For this review, take the finished solid that the model builds, in its own axes (mm). A direction names the side the tool comes from. Round coordinates to 2 decimals unless told otherwise and drop trailing zeros.
from build123d import *

# Parameters (mm, degrees)
SALIENTE_EXTRUIR1_DEPTH = 5.5
CROQUIS3_W              = 12.5
CROQUIS3_H              = 5.5
SALIENTE_EXTRUIR2_DEPTH = 25
CROQUIS6_R              = 0.88
CORTAR_EXTRUIR3_DEPTH   = 1
CORTAR_EXTRUIR4_DEPTH   = 5.75
CROQUIS7_W              = 3.3125
CROQUIS7_H              = 5.5
SALIENTE_EXTRUIR3_DEPTH = 5
SALIENTE_EXTRUIR6_DEPTH = 5.5


with BuildPart() as part:
    # Croquis2 → Saliente-Extruir1 (new body)
    with BuildSketch(Plane(origin=(0, 0, 0), x_dir=(1, 0, 0), z_dir=(0, 1, 0))):
        with BuildLine():
            Line((0, 0), (0, 12.5))
            Line((0, 12.5), (90, 36.615427319))
            add(Edge.make_bspline(
                [(0, 0), (0.391394635, 0.015775005), (1.186974035, 0.048775969), (2.973718865, 0.125104104), (4.540088904, 0.200260299), (6.566615662, 0.300718996), (8.325276336, 0.397659311), (10.239345298, 0.508699867), (12.06569896, 0.624646025), (14.401457649, 0.783062706), (17.174575564, 0.991527453), (20.424315772, 1.267095632), (24.124041131, 1.631890725), (28.746499447, 2.160588299), (34.186717026, 2.916408992), (39.59920567, 3.869463595), (44.959442778, 5.077074293), (49.361815827, 6.280418231), (52.910692092, 7.400878923), (56.408168852, 8.673928793), (59.841449897, 10.111450972), (63.196917977, 11.722972852), (66.459987179, 13.514457641), (69.616669404, 15.487724177), (72.654216734, 17.639793831), (75.562633469, 19.963554552), (78.411401775, 22.516402339), (80.637238299, 24.750127709), (82.31420302, 26.576865179), (83.500174761, 27.941909388), (84.166451521, 28.729544399), (84.824720597, 29.529498585), (85.467901785, 30.330572576), (86.10961807, 31.152932899), (86.725824802, 31.959637263), (87.359215775, 32.814913902), (87.935303716, 33.605334305), (88.585351463, 34.5293994), (89.07725637, 35.234721433), (89.639386065, 36.072003958), (89.880241627, 36.43386466), (90, 36.615427319)],
                knots=[0.074542826, 0.074542826, 0.074542826, 0.074542826, 0.074542826, 0.089942005, 0.105341185, 0.120740364, 0.136139543, 0.151538723, 0.166937902, 0.182337082, 0.197736262, 0.22853462, 0.259332978, 0.290131335, 0.320929692, 0.382526405, 0.441205382, 0.472003704, 0.502802054, 0.533600416, 0.564398766, 0.595197066, 0.625995423, 0.656793872, 0.687592091, 0.718390433, 0.749188737, 0.779987363, 0.814189109, 0.822739652, 0.831290195, 0.839840738, 0.848391281, 0.856941796, 0.865492311, 0.874042825, 0.88259334, 0.891143874, 0.899694409, 0.908244943, 0.916795477, 0.916795477, 0.916795477, 0.916795477, 0.916795477], degree=4))
        make_face()
    extrude(amount=SALIENTE_EXTRUIR1_DEPTH)

    # Croquis3 → Saliente-Extruir2 (add)
    with BuildSketch(Plane.ZY):
        with Locations((-6.25, 2.75)):
            Rectangle(CROQUIS3_W, CROQUIS3_H)
    extrude(amount=SALIENTE_EXTRUIR2_DEPTH)

    # Croquis6 → Cortar-Extruir3 (cut)
    with BuildSketch(Plane.XY):
        with Locations((-5, 2.75)):
            Circle(CROQUIS6_R)
    extrude(amount=-CORTAR_EXTRUIR3_DEPTH, mode=Mode.SUBTRACT)

    # Croquis5 → Cortar-Extruir4 (cut)
    with BuildSketch(Plane.XY):
        with BuildLine():
            Line((-25, 5.5), (-25, 0))
            Line((-25, 0), (-5.000000004, 0))
            ThreePointArc((-5.000000004, 0), (-7.75, 2.750000002), (-5, 5.5))
            Line((-5, 5.5), (-25, 5.5))
        make_face()
    extrude(amount=-CORTAR_EXTRUIR4_DEPTH, mode=Mode.SUBTRACT)

    # Croquis7 → Saliente-Extruir3 (add)
    with BuildSketch(Plane.ZY.offset(25)):
        with Locations((-10.84375, 2.75)):
            Rectangle(CROQUIS7_W, CROQUIS7_H)
    extrude(amount=SALIENTE_EXTRUIR3_DEPTH)

    # Croquis10 → Saliente-Extruir6 (add)
    with BuildSketch(Plane(origin=(0, 5.5, 0), x_dir=(1, 0, 0), z_dir=(0, 1, 0))):
        Polygon((23.606721454, 29.684431199), (26.321478766, 19.552818979), (31.634070811, 20.976323727), (29.03783695, 30.665600406), align=None)
        Polygon((81.052969303, 40.062499841), (82.514074846, 34.60957972), (87.826666891, 36.033084468), (86.484084799, 41.043669048), align=None)
    extrude(amount=-SALIENTE_EXTRUIR6_DEPTH)


solid = part.part
(1) For line 1 along Y through (x, z) = (-5, -0.35); line 2 along Z through (x, y) = (-1.5, 5.05); line 3 along Z through (x, y) = (-13.5, 3.75), list the stretches that pass through material, from the lowest coordinate up.
Geometry check:
line 1: y = 0 to 1.87, 3.63 to 5.5
line 2: z = -12.5 to 0
line 3: z = -12.5 to -5.75
(2) For faces 1 (the face through (-7.75, 2.69, -2.83)), 2 (the face through (-25, 3, -7)), 3 (the face through (24.945, 2.788, -24.69)), 4 (the face through (88.9, 2.71, -36.32)), list the 3-axis set-ups (+Z, -Z, +X, -X, +Y, -Y) from which the entire face can be reached by the end or side of a thin tool; tool diameter is ignored.
Geometry check:
face 1: +Z, -X
face 2: +Z, -X, +Y, -Y
face 3: -X, +Y, -Y
face 4: -Z, +Y, -Y
(3) Mouldability with a two-part tool opening along X and no side actions: class faces 5 (the face through (81.773, 2.788, -37.374)), 6 (the face through (30.354, 2.788, -25.753)), 7 (the face through (56.72, 2.71, -27.7)), 8 (the face through (31, 0, -16)) as pulls with the +X half, pulls with the -X half, needs draft (parallel to the pull), parting line crosses it, or undercut.
Geometry check:
face 5: pulls with the -X half
face 6: undercut
face 7: undercut
face 8: needs draft
(4) For pin 1 Ø3 at (y, z) = (1.5, -7) entering from -X; pin 2 Ø1 at (y, z) = (3.5, -34) entering from +X; pin 3 Ø2 at (y, z) = (2, -30) entering from -X; pin 4 Ø1.9 at (x, y) = (-5, 3) entering from +Z, all flat-tipped, find the tip position at first contact; note any pin that passes through.
Geometry check:
pin 1: stops at x = -25
pin 2: stops at x = 88.56
pin 3: stops at x = 23.61
pin 4: stops at z = 0
